```python
from build123d import *

# Parameters (mm, degrees)
F0_R     = 25
F0_R_2   = 12.5
F1_DEPTH = 100
F2_SIZE  = 5
F3_SIZE  = 5
F5_D     = 5.5
F5_DEPTH = 25.001


with BuildPart() as f1:
    # F0 (on Top) → F1 (new body)
    with BuildSketch(Plane.XY):
        Circle(F0_R)
        Circle(F0_R_2, mode=Mode.SUBTRACT)
    extrude(amount=F1_DEPTH)

    # F2
    f2_edges = [f1.edges().sort_by_distance(p)[0] for p in [
        (-25, 0, 100),
    ]]
    chamfer(f2_edges, length=F2_SIZE)

    # F3
    f3_edges = [f1.edges().sort_by_distance(p)[0] for p in [
        (-25, 0, 0),
    ]]
    chamfer(f3_edges, length=F3_SIZE)

    # F5 (through all, one way)
    with BuildSketch(Plane(origin=(0, 0, 0), x_dir=(1, 0, 0), z_dir=(0, 1, 0))):
        with Locations((0, -35)):
            Circle(F5_D / 2)
    extrude(amount=-F5_DEPTH, mode=Mode.SUBTRACT)


solid = f1.part
```
The listing builds one solid part. Answer for the finished solid, in the listing's coordinates (mm). A direction names the side the tool comes from. Coordinates: 2 decimals unless noted, no trailing zeros. Write each loop counter-clockwise with the first axis right and the second up, starting at its lowest first coordinate (ties: lowest second). Pieces come first, ordered by that corner, then holes. Notation, with made-up numbers: M -15.5,-2.75 L -10.5,-2.75 A6 ccw -10.5,4.25 Z; hole C -29.5,82.5 d6. An arc over 180 degrees is marked long. Use a Markdown table: item, result. Add a question column.
1. Straight lines are drawn through the part: line 1 along Z through (x, y) = (0, -17); line 2 along Y through (x, z) = (9, 5); line 3 along X through (y, z) = (6, 34.5). For each, find the intervals that lie inside material, in ascending order. Write a range as [from, to].
2. Section B-B (x = 0) is taken. Give the vertices of the cut face in (y, z).
3. Section C-C (z = 20.5) is taken. Give the vertices of the cut face in (x, y), plus the area to 3 significant figures.
4. Which of the six approach directions +Z, -Z, +X, -X, +Y, -Y give full straight-line access (tool end or side, diameter ignored) to faces 1 (the cylindrical face through (23.846, 7.509, 49.37)), 2 (the cylindrical face through (-0.358, -18.508, 32.273))?
5. For a pull along X with two mould halves and no side action, classify faces 3 (the conical face through (-4.39, -19.76, 0.24)), 4 (the flat face through (-9, -9, 100)), 5 (the cylindrical face through (11.923, 3.755, 49.3)) as +X half, -X half, draft (parallel to the pull), parting line (faces both ways), or undercut.
6. Given P1, Ø6, axis at y = -18, z = 13.5, coming from the +X side; P2, Ø5, axis at x = 0, z = 34, coming from the +Y side; P3, Ø1, axis at x = 4, z = 71.5, coming from the +Y side; P4, Ø10, axis at x = 4, y = 10.5, coming from the -Z side, each flat-ended and moving along its own axis, determine where each tip first touches the part or whether it passes through.
7. Section A-A (y = 0) is taken. Give the vertices of the cut face in (x, z).
8. Section D-D (z = 35) is taken. Give the vertices of the cut face in (x, y).
Data:
| question | item | result |
|---|---|---|
| 1 | line 1 | z = [0, 32.25], [37.75, 100] |
| 1 | line 2 | y = [-23.32, -8.67], [8.67, 23.32] |
| 1 | line 3 | x = [-24.27, -10.97], [10.97, 24.27] |
| 2 | outline | M -25,5 L -20,0 L -12.5,0 L -12.5,32.25 L -25,32.25 Z; M -25,37.75 L -12.5,37.75 L -12.5,100 L -20,100 L -25,95 Z; M 12.5,0 L 20,0 L 25,5 L 25,95 L 20,100 L 12.5,100 Z |
| 3 | outline | C 0,0 d50; hole C 0,0 d25 |
| 3 | area | 1,470 mm2 |
| 4 | face 1 | +Z, -Z |
| 4 | face 2 | -Y |
| 5 | face 3 | parting line |
| 5 | face 4 | draft |
| 5 | face 5 | undercut |
| 6 | P1 | stops at x = 20 |
| 6 | P2 | stops at y = 25 |
| 6 | P3 | stops at y = 24.75 |
| 6 | P4 | stops at z = 0 |
| 7 | outline | M -25,5 L -20,0 L -12.5,0 L -12.5,100 L -20,100 L -25,95 Z; M 12.5,0 L 20,0 L 25,5 L 25,95 L 20,100 L 12.5,100 Z |
| 8 | outline | M -2.75,-24.85 L -2.75,-12.19 A12.5 cw long 2.75,-12.19 L 2.75,-24.85 A25 ccw long Z |
